Source: CAD feature listing. Evaluate the final solid. Frame: model axes, mm. Face numbers are marked on the shaded views. A direction names the side the tool comes from. Give positions to 0.01 mm unless a question says otherwise; leave off trailing zeros. Order: outer loops, then holes, each group sorted by start corner. A loop starts at its lowest first (then second) coordinate and runs counter-clockwise, first axis right, second up.
1) First-contact query: P1, Ø5, axis at x = 2, z = -13.5, coming from the -Y side (3 decimals); P2, Ø4, axis at x = 0.5, z = 3.5, coming from the +Y side; P3, Ø3, axis at x = 0.5, y = -0.5, coming from the +Z side; P4, Ø3, axis at y = 1.5, z = -11, coming from the +X side (3 decimals). Flat tips, straight axial feed; report the tip coordinate or a pass-through.
2) Draft query along Y for the marked faces 3, 4 and 5. Return one class per face: released by +Y, released by -Y, zero draft, split by the parting line, or undercut.
3) Material intervals for line 1 (Z direction, x = 4.25, y = 1.25); line 2 (Y direction, x = -2, z = 3.75); line 3 (X direction, y = 0.5, z = 1.5), sorted ascending.
4) Access query for the marked faces 1 and 2. Directions: +Z, -Z, +X, -X, +Y, -Y. A direction counts if a zero-diameter tool reaches every point of the face in a straight line with its end or side. Return the directions, or none.
5) Section B-B, the plane z = -9.25. Return loops of the section in (x, y) (3 decimals).
6) Section A-A, the plane x = 0. Return loops of the section in (y, z) (3 decimals), plus the area to 3 significant figures.
Solid Edge part; units mm, degrees
sketch "Sketch1" plane through (0, 0, 0) normal (0, 0, 1) x (1, 0, 0)
  circle A0 centre (0, 0) radius 3.175
extrude "Protrusion1" add sketch "Sketch1" against normal blind 25
sketch "Sketch2" plane through (0, 0, 0) normal (0, 0, 1) x (1, 0, 0)
  circle A0 centre (0, 0) radius 5
extrude "ExtrudedProtrusion_2" add sketch "Sketch2" along normal blind 5
fillet "Round_1" radius 0.5 2 edges at (-5, 0, 5) (-5, 0, 0)
sketch "Sketch3" plane through (0, 0, 5) normal (0, 0, 1) x (1, 0, 0)
  line L0 (-1.7321, 3) -> (-3.4641, 0)
  line L1 (-3.4641, 0) -> (-1.7321, -3)
  line L2 (-1.7321, -3) -> (1.7321, -3)
  line L3 (1.7321, -3) -> (3.4641, 0)
  line L4 (3.4641, 0) -> (1.7321, 3)
  line L5 (1.7321, 3) -> (-1.7321, 3)
extrude "ExtrudedCutout_1" cut sketch "Sketch3" against normal blind 4
chamfer "Chamfer_1" distance 0.5 angle 45 1 edges at (-3.175, 0, -25) measured on face at (-2.1802, -2.0532, -25)
cosmetic_thread "Thread1"
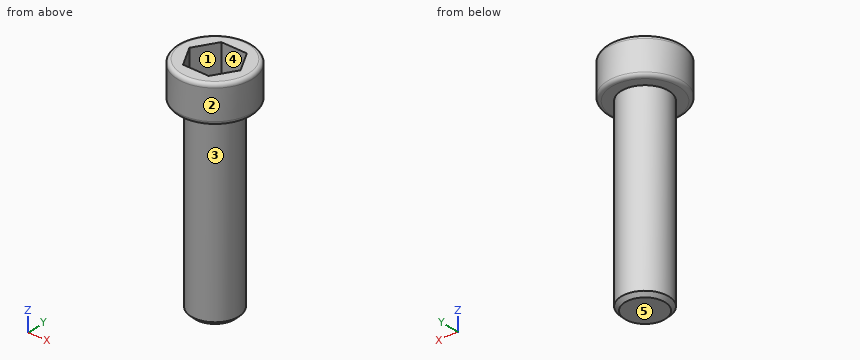
From the geometry:
1. P1: stops at y = -3.175
1. P2: stops at y = 5
1. P3: stops at z = 1
1. P4: stops at x = 3.175
2. face 3: split by the parting line
2. face 4: undercut
2. face 5: zero draft
3. line 1: z = 0 to 5
3. line 2: y = -4.58 to -2.54, 2.54 to 4.58
3. line 3: x = -4.97 to -3.18, 3.18 to 4.97
4. face 1: +Z
4. face 2: +Z, -Z
5. outline: circle Ø6.35 at (0, 0)
6. outline: (-5, 0.5) arc R0.5 ccw to (-4.5, 0) - (-3.175, 0) - (-3.175, -24.5) - (-2.675, -25) - (2.675, -25) - (3.175, -24.5) - (3.175, 0) - (4.5, 0) arc R0.5 ccw to (5, 0.5) - (5, 4.5) arc R0.5 ccw to (4.5, 5) - (3, 5) - (3, 1) - (-3, 1) - (-3, 5) - (-4.5, 5) arc R0.5 ccw to (-5, 4.5) - close
6. area: 184 mm2
